from build123d import *

# Parameters (mm, degrees)
SKETCH1_W           = 92.71
SKETCH1_H           = 92.71
SKETCH1_R           = 5.3578125
BOSS_EXTRUDE1_DEPTH = 6.35
SKETCH2_R           = 1.4224
CUT_EXTRUDE1_DEPTH  = 6.35


with BuildPart() as part:
    # Sketch1 → Boss-Extrude1 (new body)
    with BuildSketch(Plane.XY):
        with Locations((46.355, 46.355)):
            Rectangle(SKETCH1_W, SKETCH1_H)
        with Locations((46.355, 46.355)):
            Circle(SKETCH1_R, mode=Mode.SUBTRACT)
    extrude(amount=BOSS_EXTRUDE1_DEPTH)

    # Sketch2 → Cut-Extrude1 (cut)
    with BuildSketch(Plane.XY.offset(6.35)):
        with Locations((2.54, 20.100036)):
            Circle(SKETCH2_R)
        with Locations((20.100036, 2.54)):
            Circle(SKETCH2_R)
        with Locations((72.609964, 2.54)):
            Circle(SKETCH2_R)
        with Locations((90.17, 20.100036)):
            Circle(SKETCH2_R)
        with Locations((90.17, 72.609964)):
            Circle(SKETCH2_R)
        with Locations((72.609964, 90.17)):
            Circle(SKETCH2_R)
        with Locations((20.100036, 90.17)):
            Circle(SKETCH2_R)
        with Locations((2.54, 72.609964)):
            Circle(SKETCH2_R)
    extrude(amount=-CUT_EXTRUDE1_DEPTH, mode=Mode.SUBTRACT)


solid = part.part
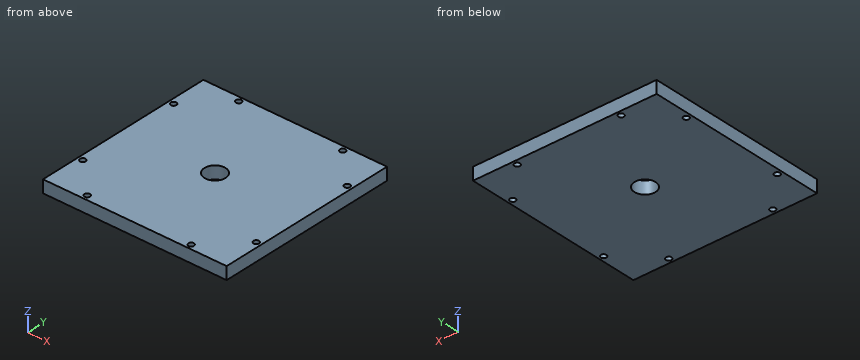
Model file for the job. Use its own axes, mm. Round coordinates to 2 decimals unless told otherwise and drop trailing zeros. Order: outer loops, then holes, each group sorted by start corner. A loop starts at its lowest first (then second) coordinate and runs counter-clockwise, first axis right, second up.
(1) Band-saw the part on D-D (x = 49.5). List the corners of the cut face in (y, z).
(2) Band-saw the part on A-A (x = 2.54). List the corners of the cut face in (y, z).
(3) Pin check, flat tips, straight feed: pin 1 (3.5 mm diameter, centred on x = 90.17, y = 20.1, fed in from +Z); pin 2 (1.7 mm diameter, centred on x = 20.1, y = 90.17, fed in from -Z). Stop position of each tip, or through.
(4) Drill centre lines: line 1 (Y direction, x = 2.54, z = 2.75); line 2 (X direction, y = 89, z = 1); line 3 (Y direction, x = 19, z = 0.5). Where is each one in solid material? Low to high.
(5) Band-saw the part on C-C (z = 2). Give the number of separate pieces and of enclosed holes in the cut face, then the cut area to 3 significant figures.
Verdict:
1. outline: (0, 0) - (42.02, 0) - (42.02, 6.35) - (0, 6.35) - close; (50.69, 0) - (92.71, 0) - (92.71, 6.35) - (50.69, 6.35) - close
2. outline: (0, 0) - (18.68, 0) - (18.68, 6.35) - (0, 6.35) - close; (21.52, 0) - (71.19, 0) - (71.19, 6.35) - (21.52, 6.35) - close; (74.03, 0) - (92.71, 0) - (92.71, 6.35) - (74.03, 6.35) - close
3. pin 1: stops at z = 6.35
3. pin 2: passes through
4. line 1: y = 0 to 18.68, 21.52 to 71.19, 74.03 to 92.71
4. line 2: x = 0 to 19.29, 20.91 to 71.8, 73.42 to 92.71
4. line 3: y = 0 to 1.64, 3.44 to 89.27, 91.07 to 92.71
5. separate pieces: 1
5. enclosed holes: 9
5. area: 8,450 mm2
